Work out the finished part from the listing and answer in its coordinate system (mm). A direction names the side the tool comes from. Round coordinates to 2 decimals unless told otherwise and drop trailing zeros. Order: outer loops, then holes, each group sorted by start corner. A loop starts at its lowest first (then second) coordinate and runs counter-clockwise, first axis right, second up. Notation, with made-up numbers: (16, 40) - (21, 40) arc R10 ccw to (21, 46) - close; hole circle Ø8 at (84, 43). An arc over 180 degrees is marked (long way). Use one line per item in the form item = value. Start each with the question number.
Q1. The part is cut by section C-C on z = -0.5. State how many separate pieces and enclosed holes the cut face has, plus the area to 3 significant figures.
Q2. Which of the six approach directions +Z, -Z, +X, -X, +Y, -Y give full straight-line access (tool end or side, diameter ignored) to faces 4 (the flat face through (154, 1, 0)), 5 (the cylindrical face through (228.361, -33.085, -1.521))?
Q3. The part is cut by section A-A on y = -7.5. Determine the outline of the cut face in (x, z), plus the area to 3 significant figures.
Q4. Given P1, Ø0.9, axis at x = -1.5, z = -1, coming from the +Y side; P2, Ø2, axis at x = 218, y = -35, coming from the -Z side; P3, Ø5, axis at x = -9, y = 0, coming from the -Z side; P4, Ø1.5, axis at x = 290, z = -2, coming from the +Y side, each flat-ended and moving along its own axis, determine where each tip first touches the part or whether it passes through.
Q5. For a pull along Y with two mould halves and no side action, classify faces 1 (the flat face through (264.56, -37.046, -1.479)), 2 (the cylindrical face through (228.19, 32.96, -1.52)), 3 (the flat face through (-10.26, 12.51, -1.48)) as +Y half, -Y half, draft (parallel to the pull), parting line (faces both ways), or undercut.
Q6. Find the intervals of material crossed by line 1 (X direction, y = -17, z = -1) (3 decimals); line 2 (Y direction, x = 2, z = -0.95); line 3 (Y direction, x = 288, z = -1.5), in increasing order. Write a range as [from, to].
Q7. The part is cut by section B-B on y = 10.5. Determine the outline of the cut face in (x, z).
Autodesk Inventor part; units mm, degrees
ref_plane "Bottom" through (0, 0, -3) normal (0, 0, 1) x (1, 0, 0)
ref_plane "5mm Inside" through (0, 0, 6) normal (0, 0, 1) x (1, 0, 0)
ref_plane "YZ Plane" through (0, 0, 0) normal (1, 0, 0) x (0, 1, 0)
sketch "Sketch1" plane through (0, 0, 0) normal (0, 0, 1) x (1, 0, 0)
  line L0 (0, 0) -> (327, 0)
  line L1 (0, 0) -> (0, -26) construction
  line L2 (0, -26) -> (60, -26)
  line L3 (60, -26) -> (81, -58)
  line L4 (81, -58) -> (215, -58)
  line L5 (215, -58) -> (260, -44)
  line L6 (260, -44) -> (270, -28.75)
  line L7 (270, -28.75) -> (310, -28.75)
  line L8 (310, -28.75) -> (324, -24)
  line L9 (324, -24) -> (327, 0)
  line L10 (0, 26) -> (60, 26)
  line L11 (60, 26) -> (81, 58)
  line L12 (81, 58) -> (215, 58)
  line L13 (215, 58) -> (260, 44)
  line L14 (260, 44) -> (270, 28.75)
  line L15 (270, 28.75) -> (310, 28.75)
  line L16 (310, 28.75) -> (324, 24)
  line L17 (324, 24) -> (327, 0)
  line L18 (0, -26) -> (0, 26)
  line L19 (0, -23.75) -> (-6, -23.75)
  line L20 (-6, -23.75) -> (-15, 0)
  line L21 (-15, 0) -> (-6, 23.75)
  line L22 (-6, 23.75) -> (0, 23.75)
  line L23 (256.5, -27.5) -> (256.5, 27.5)
  line L24 (256.5, 27.5) -> (225, 37.5)
  line L25 (225, 37.5) -> (225, -37.5)
  line L26 (225, -37.5) -> (256.5, -27.5)
  point P0 (-9, 0)
  point P1 (0, 0)
  point P2 (-3, -19.75)
  point P3 (11, -18.5)
  point P4 (64, -13)
  point P5 (145, -35)
  point P6 (218, -35)
  point P7 (218, -19)
  point P8 (261, -19)
  point P9 (317, -19)
  point P10 (224, -51)
  dimension "d1" = 26
  dimension "d2" = 60
  dimension "d3" = 58
  dimension "d4" = 28.75
  dimension "d6" = 24
  dimension "d9" = 44
  dimension "d15" = 15
  dimension "d16" = 6
  dimension "d19" = 47.5
  dimension "d20" = 256.5
  dimension "d21" = 75
  dimension "d22" = 55
  dimension "d23" = 31.5
  dimension "d24" = 81
  dimension "d25" = 215
  dimension "d26" = 260
  dimension "d27" = 270
  dimension "d28" = 310
  dimension "d29" = 324
  dimension "d30" = 327
  dimension "d190" = 9
  dimension "d191" = 3
  dimension "d192" = 4
  dimension "d193" = 7.5
  dimension "frhole0" = 11
  dimension "d195" = 13
  dimension "d196" = 64
  dimension "d197" = 23
  dimension "d198" = 145
  dimension "d199" = 73
  dimension "RF_Bulkhead" = 43
  dimension "RR_Bulkhead" = 56
  dimension "d242" = 1
  dimension "d243" = 7
  dimension "d244" = 7
  dimension "d245" = 39
ref_plane "Bottom" through (0, 0, -3) normal (0, 0, 1) x (1, 0, 0)
sketch "Hole_Centres" plane through (0, 0, -3) normal (0, 0, 1) x (1, 0, 0)
  point P0 (-9, 0)
  point P1 (-3, -19.75)
  point P2 (11, -18.5)
  point P3 (64, -13)
  point P4 (145, -35)
  point P5 (218, -19)
  point P6 (224, -51)
  point P7 (261, -19)
  point P8 (317, -19)
  point P9 (218, -35)
  point P10 (37, -18.5)
  point P11 (71, -18.5)
  dimension "frhole1" = 26
  dimension "frhole2" = 34
extrude "Extrusion1" add sketch "Sketch1" against normal blind 3
fillet "Fillet1" radius 8 14 edges at (60, 26, -1.5) (60, -26, -1.5) (81, -58, -1.5) (215, -58, -1.5) (260, -44, -1.5) (270, -28.75, -1.5) (260, 44, -1.5) (215, 58, -1.5) (81, 58, -1.5) (310, -28.75, -1.5) (310, 28.75, -1.5) (327, 0, -1.5) (-15, 0, -1.5) (270, 28.75, -1.5)
fillet "Fillet2" radius 2 4 edges at (-6, -23.75, -1.5) (-6, 23.75, -1.5) (324, -24, -1.5) (324, 24, -1.5)
ref_plane "5mm Inside" through (0, 0, 6) normal (0, 0, 1) x (1, 0, 0)
extrude "Extrusion10" cut sketch "Sketch1" along normal through all both and the other way through all contours L25 L24 L23 L0 | L0 L23 L26 L25
fillet "Fillet9" radius 8 4 edges at (225, -37.5, -1.5) (225, 37.5, -1.5) (256.5, 27.5, -1.5) (256.5, -27.5, -1.5)
hole "Hole2" at (-3, -19.75, -3) at (11, -18.5, -3) at (145, -35, -3) at (218, -19, -3) at (224, -51, -3) at (261, -19, -3) at (317, -19, -3) at (218, -35, -3) at (37, -18.5, -3) at (71, -18.5, -3) direction (0, 0, 1) diameter 3.4 end through all countersink diameter 6.3 countersink angle 90
mirror "Mirror6" about plane through (0, 0, 0) normal (0, 1, 0) of "Hole2"
hole "Hole3" at (-9, 0, -3) direction (0, 0, 1) diameter 3 end through all countersink diameter 6 countersink angle 90
equation "\"d99\" = d43"
equation "\"d101\" = d31"
properties part number "WSC2011_TP05_01_CHASSIS" material "ABS Plastic"
Found:
q1.separate_pieces = 1
q1.enclosed_holes = 22
q1.area = 27,200 mm²
q2.face_4 = +Z, +X, -X, +Y, -Y
q2.face_5 = +Z, -Z
q3.outline = (-12.16, -3) - (225, -3) - (225, 0) - (-12.16, 0) - close; (256.5, -3) - (326.06, -3) - (326.06, 0) - (256.5, 0) - close
q3.area = 920 mm²
q4.P1 = 23.75
q4.P2 = through
q4.P3 = -2.5
q4.P4 = 28.75
q5.face_1 = -Y half
q5.face_2 = undercut
q5.face_3 = +Y half
q6.line_1 = [-8.558, 10.2], [11.8, 36.2], [37.8, 70.2], [71.8, 225], [256.5, 324.875]
q6.line_2 = [-26, 26]
q6.line_3 = [-28.75, 28.75]
q7.outline = (-11.02, -3) - (225, -3) - (225, 0) - (-11.02, 0) - close; (256.5, -3) - (325.69, -3) - (325.69, 0) - (256.5, 0) - close
